Geometry: final body of the model. Coordinates: model frame, mm. Coordinates: 2 decimals unless noted, no trailing zeros. Order: outer loops, then holes, each group sorted by start corner. A loop starts at its lowest first (then second) coordinate and runs counter-clockwise, first axis right, second up. Notation, with made-up numbers: (-27, 27) -> (15, 27) arc R22 cw to (15, 55) -> close; hole circle Ø6 at (62, -14.5). An arc over 180 degrees is marked (long way). Use one line per item in the form item = value.
```python
from build123d import *

# Parameters (mm, degrees)
F0_W     = 50
F0_H     = 70
F1_DEPTH = 3
F3_D     = 3
F6_DEPTH = 33


with BuildPart() as f1:
    # F0 (on Top) → F1 (new body)
    with BuildSketch(Plane.XY):
        with Locations((25, 35)):
            Rectangle(F0_W, F0_H)
    extrude(amount=F1_DEPTH)

    # F3 (through all)
    with Locations(Plane.XY.offset(3)):
        with Locations((35, 20), (35, 60)):
            Hole(F3_D / 2)

    # F5 (on face) → F6 (cut)
    with BuildSketch(Plane.XY.offset(3)):
        with BuildLine():
            ThreePointArc((44.21057, 59.963956), (41.71057, 62.463956), (39.21057, 59.963956))
            Line((39.21057, 59.963956), (39.21057, 14.963956))
            ThreePointArc((39.21057, 14.963956), (41.71057, 12.463956), (44.21057, 14.963956))
            Line((44.21057, 14.963956), (44.21057, 59.963956))
        make_face()
    extrude(amount=-F6_DEPTH, mode=Mode.SUBTRACT)

    # F7: F1 across plane


with BuildPart() as f1_1:
    add(f1.part)
    add(f1.part.mirror(Plane.XY))

    # F8: F1 across plane


with BuildPart() as f1_2:
    add(f1_1.part)
    add(f1_1.part.mirror(Plane.YZ))


solid = f1_2.part
```
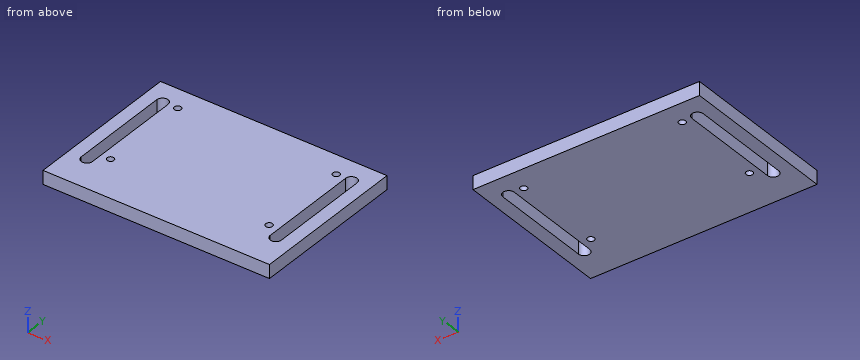
1) Section D-D, the plane z = -0.8. Output: boundary loops of the cut face in (x, y).
Results found:
outline = (-50, 0) -> (50, 0) -> (50, 70) -> (-50, 70) -> close; hole (-44.21, 14.96) arc R2.5 ccw to (-39.21, 14.96) -> (-39.21, 59.96) arc R2.5 ccw to (-44.21, 59.96) -> close; hole circle Ø3 at (-35, 20); hole circle Ø3 at (-35, 60); hole circle Ø3 at (35, 20); hole circle Ø3 at (35, 60); hole (39.21, 14.96) arc R2.5 ccw to (44.21, 14.96) -> (44.21, 59.96) arc R2.5 ccw to (39.21, 59.96) -> close
2) Contact query for flat-ended pins moving along their axis: P1, Ø1.8, axis at x = 35, y = 60, coming from the +Z side; P2, Ø1, axis at x = -10.5, z = -0.5, coming from the -Y side. Output: stop coordinate, or through.
Results found:
P1 = through
P2 = 0
3) Section C-C, the plane x = 35. Output: boundary loops of the cut face in (y, z).
Results found:
outline = (0, -3) -> (18.5, -3) -> (18.5, 3) -> (0, 3) -> close; (21.5, -3) -> (58.5, -3) -> (58.5, 3) -> (21.5, 3) -> close; (61.5, -3) -> (70, -3) -> (70, 3) -> (61.5, 3) -> close
4) Section B-B, the plane y = 20. Output: boundary loops of the cut face in (x, z), and give its area (3 significant figures).
Results found:
outline = (-50, -3) -> (-44.21, -3) -> (-44.21, 3) -> (-50, 3) -> close; (-39.21, -3) -> (-36.5, -3) -> (-36.5, 3) -> (-39.21, 3) -> close; (-33.5, -3) -> (33.5, -3) -> (33.5, 3) -> (-33.5, 3) -> close; (36.5, -3) -> (39.21, -3) -> (39.21, 3) -> (36.5, 3) -> close; (44.21, -3) -> (50, -3) -> (50, 3) -> (44.21, 3) -> close
area = 504 mm2
5) Material intervals for probe 1 along X at (y, z) = (36, 1.7); probe 2 along Y at (x, z) = (35, 1.3); probe 3 along X at (y, z) = (62, 1.45), sorted ascending. Write a range as from..to.
Results found:
probe_1 = -50..-44.21, -39.21..39.21, 44.21..50
probe_2 = 0..18.5, 21.5..58.5, 61.5..70
probe_3 = -50..-43.16, -40.26..40.26, 43.16..50
6) Section A-A, the plane y = 28. Output: boundary loops of the cut face in (x, z), and give its area (3 significant figures).
Results found:
outline = (-50, -3) -> (-44.21, -3) -> (-44.21, 3) -> (-50, 3) -> close; (-39.21, -3) -> (39.21, -3) -> (39.21, 3) -> (-39.21, 3) -> close; (44.21, -3) -> (50, -3) -> (50, 3) -> (44.21, 3) -> close
area = 540 mm2
